```python
from build123d import *

# Parameters (mm, degrees)
BOSS_EXTRUDE1_DEPTH = 5
CUT_EXTRUDE1_DEPTH  = 10
CUT_EXTRUDE2_DEPTH  = 10
SKETCH5_W           = 5
SKETCH5_H           = 43.988909765
CUT_EXTRUDE4_DEPTH  = 5
CUT_EXTRUDE6_DEPTH  = 10
SKETCH8_W           = 43
SKETCH8_H           = 10
CUT_EXTRUDE7_DEPTH  = 10


with BuildPart() as part:
    # Sketch1 → Boss-Extrude1 (new body)
    with BuildSketch(Plane.XY):
        with BuildLine():
            Line((100, 25), (85, 25))
            ThreePointArc((85, 25), (83.205104603, 25.333271969), (81.649484536, 26.288659794))
            Line((81.649484536, 26.288659794), (51.958762887, 53.092783505))
            Line((51.958762887, 53.092783505), (55.309278351, 56.804123711))
            Line((55.309278351, 56.804123711), (33.041237113, 76.907216495))
            Line((33.041237113, 76.907216495), (29.690721649, 73.195876289))
            Line((29.690721649, 73.195876289), (7.422680412, 93.298969072))
            Line((7.422680412, 93.298969072), (0, 85.076923077))
            Line((0, 85.076923077), (0, 0))
            Line((0, 0), (30, 0))
            Line((30, 0), (30, -5))
            Line((30, -5), (65, -5))
            Line((65, -5), (65, 0))
            Line((65, 0), (165, 0))
            Line((165, 0), (165, -5))
            Line((165, -5), (200, -5))
            Line((200, -5), (200, 0))
            Line((200, 0), (230, 0))
            Line((230, 0), (230, 85.076923077))
            Line((230, 85.076923077), (222.577319588, 93.298969072))
            Line((222.577319588, 93.298969072), (200.309278351, 73.195876289))
            Line((200.309278351, 73.195876289), (196.958762887, 76.907216495))
            Line((196.958762887, 76.907216495), (174.690721649, 56.804123711))
            Line((174.690721649, 56.804123711), (178.041237113, 53.092783505))
            Line((178.041237113, 53.092783505), (148.350515464, 26.288659794))
            ThreePointArc((148.350515464, 26.288659794), (146.794895397, 25.333271969), (145, 25))
            Line((145, 25), (130, 25))
            Line((130, 25), (130, 30))
            Line((130, 30), (100, 30))
            Line((100, 30), (100, 25))
        make_face()
    extrude(amount=BOSS_EXTRUDE1_DEPTH)

    # Sketch2 → Cut-Extrude1 (cut)
    with BuildSketch(Plane(origin=(0, 0, 0), x_dir=(-1, 0, 0), z_dir=(0, 0, -1))):
        Polygon((0, 25), (0, 0), (-25, 0), align=None)
        Polygon((-230, 0), (-205, 0), (-230, 25), align=None)
    extrude(amount=-CUT_EXTRUDE1_DEPTH, mode=Mode.SUBTRACT)

    # Sketch3 → Cut-Extrude2 (cut)
    with BuildSketch(Plane(origin=(0, 0, 0), x_dir=(-1, 0, 0), z_dir=(0, 0, -1))):
        with BuildLine():
            Line((-82, 7.5), (-93.5, 7.5))
            ThreePointArc((-93.5, 7.5), (-94.914213562, 8.085786438), (-95.5, 9.5))
            Line((-95.5, 9.5), (-95.5, 15.5))
            ThreePointArc((-95.5, 15.5), (-94.914213562, 16.914213562), (-93.5, 17.5))
            Line((-93.5, 17.5), (-82, 17.5))
            ThreePointArc((-82, 17.5), (-80.585786438, 16.914213562), (-80, 15.5))
            Line((-80, 15.5), (-80, 9.5))
            ThreePointArc((-80, 9.5), (-80.585786438, 8.085786438), (-82, 7.5))
        make_face()
        with BuildLine():
            Line((-134.5, 9.5), (-134.5, 15.5))
            ThreePointArc((-134.5, 15.5), (-135.085786438, 16.914213562), (-136.5, 17.5))
            Line((-136.5, 17.5), (-148, 17.5))
            ThreePointArc((-148, 17.5), (-149.414213562, 16.914213562), (-150, 15.5))
            Line((-150, 15.5), (-150, 9.5))
            ThreePointArc((-150, 9.5), (-149.414213562, 8.085786438), (-148, 7.5))
            Line((-148, 7.5), (-136.5, 7.5))
            ThreePointArc((-136.5, 7.5), (-135.085786438, 8.085786438), (-134.5, 9.5))
        make_face()
    extrude(amount=-CUT_EXTRUDE2_DEPTH, mode=Mode.SUBTRACT)

    # Sketch5 → Cut-Extrude4 (cut)
    with BuildSketch(Plane(origin=(12.5, 12.5, 0), x_dir=(0, 0, 1), z_dir=(-0.707106781, -0.707106781, 0))):
        with Locations((2.5, 0.781251447)):
            Rectangle(SKETCH5_W, SKETCH5_H)
    cut_extrude4 = extrude(amount=-CUT_EXTRUDE4_DEPTH, mode=Mode.SUBTRACT)

    # Mirror1: Cut-Extrude4 across plane
    add(cut_extrude4.mirror(Plane(origin=(115, 0, 0), x_dir=(0, 0, 1), z_dir=(1, 0, 0))), mode=Mode.SUBTRACT)

    # Sketch7 → Cut-Extrude6 (cut)
    with BuildSketch(Plane(origin=(0, 0, 0), x_dir=(-1, 0, 0), z_dir=(0, 0, -1))):
        Polygon((-23.086143571, 16.055992052), (-21.035533906, 18.106601718), (-18.065685425, 21.076450199), (-16.01507576, 23.127059864), (-23.086143571, 30.198127676), (-30.157211383, 23.127059864), align=None)
        Polygon((-21.035533906, 18.106601718), (-17.5, 14.571067812), (-14.530151519, 17.540916293), (-18.065685425, 21.076450199), align=None)
        Polygon((-213.98492424, 23.127059864), (-206.913856429, 30.198127676), (-199.842788617, 23.127059864), (-206.913856429, 16.055992052), align=None)
        Polygon((-208.964466094, 18.106601718), (-211.934314575, 21.076450199), (-215.469848481, 17.540916293), (-212.5, 14.571067812), align=None)
    extrude(amount=-CUT_EXTRUDE6_DEPTH, mode=Mode.SUBTRACT)

    # Sketch8 → Cut-Extrude7 (cut)
    with BuildSketch(Plane(origin=(0, 0, 0), x_dir=(-1, 0, 0), z_dir=(0, 0, -1))):
        with Locations((-115, 12.5)):
            Rectangle(SKETCH8_W, SKETCH8_H)
    extrude(amount=-CUT_EXTRUDE7_DEPTH, mode=Mode.SUBTRACT)


solid = part.part
```
Could you check a few things on this model? Use its own coordinates, in mm. A direction names the side the tool comes from. Coordinates: 2 decimals unless noted, no trailing zeros. Order: outer loops, then holes, each group sorted by start corner. A loop starts at its lowest first (then second) coordinate and runs counter-clockwise, first axis right, second up. Notation, with made-up numbers: M 9.5,67.25 L 36.5,67.25 A16 cw 36.5,75.25 Z; hole C -26.5,-26 d5. An arc over 180 degrees is marked long. Use a Markdown table: item, result. Add a question column.
Q1. I want a section at C-C on x = 160. List the corners of the cut face in (y, z) for me, then the cut area to 3 significant figures.
Q2. I want a section at A-A on y = 87.5. List the corners of the cut face in (x, z) for me, then the cut area to 3 significant figures.
Q3. If I drill on L1, parallel to Y at x = 84.5, z = 0.85; L2, parallel to X at y = 74.5, z = 4.8; L3, parallel to X at y = 18, z = 2.2, over which ranges is the centre line in solid material (lowest first)?
Q4. Which directions (+Z, -Z, +X, -X, +Y, -Y) give clear straight access to the entire face, cutting with the end or side of a thin tool? Please do faces 1 (the flat face through (30, -2, 2)), 2 (the flat face through (200, -3, 2)), 3 (the flat face through (80, 13, 2)), 4 (the flat face through (165, -2, 2)), 5 (the flat face through (93, 25, 2)).
Q5. I want a section at B-B on y = 68. List the corners of the cut face in (x, z) for me, then the cut area to 3 significant figures.
Q6. I'm going to push flat-ended pins straight in: pin 1 (2.5 mm diameter, centred on y = 13, z = 3, fed in from +X); pin 2 (1.5 mm diameter, centred on x = 110.5, z = 3.5, fed in from -Y); pin 3 (2.5 mm diameter, centred on y = 28.5, z = 2, fed in from +X). Where does each tip first touch, or does it pass through?
Q7. I want a section at D-D on x = 62. List the corners of the cut face in (y, z) for me, then the cut area to 3 significant figures.
Checked values:
| question | item | result |
|---|---|---|
| 1 | outline | M 0,0 L 36.81,0 L 36.81,5 L 0,5 Z |
| 1 | area | 184 mm² |
| 2 | outline | M 2.19,0 L 13.85,0 L 13.85,5 L 2.19,5 Z; M 216.15,0 L 227.81,0 L 227.81,5 L 216.15,5 Z |
| 2 | area | 117 mm² |
| 3 | L1 | 0 to 7.5, 17.5 to 25.03 |
| 3 | L2 | 0 to 28.25, 30.87 to 35.71, 194.29 to 199.13, 201.75 to 230 |
| 3 | L3 | 14.07 to 14.99, 20.93 to 21.14, 25.03 to 204.97, 208.86 to 209.07, 215.01 to 215.93 |
| 4 | face 1 | +Z, -Z, -X, -Y |
| 4 | face 2 | +Z, -Z, +X, -Y |
| 4 | face 3 | +Z, -Z |
| 4 | face 4 | +Z, -Z, -Y |
| 4 | face 5 | +Z, -Z, +Y |
| 5 | outline | M 0,0 L 42.91,0 L 42.91,5 L 0,5 Z; M 187.09,0 L 230,0 L 230,5 L 187.09,5 Z |
| 5 | area | 429 mm² |
| 6 | pin 1 | x = 212.18 |
| 6 | pin 2 | y = 0 |
| 6 | pin 3 | x = 227.68 |
| 7 | outline | M -5,0 L 44.03,0 L 44.03,5 L -5,5 Z |
| 7 | area | 245 mm² |
